Design review of the part built by this model. Coordinates are the model's own, in mm. A direction names the side the tool comes from. Give positions to 0.01 mm unless a question says otherwise; leave off trailing zeros. Write each loop counter-clockwise with the first axis right and the second up, starting at its lowest first coordinate (ties: lowest second). Pieces come first, ordered by that corner, then holes.
Autodesk Inventor part; units mm, degrees
ref_plane "Work Plane1" through (-9.8235, 15.24, 1.6002) normal (0, 1, 0) x (1, 0, 0)
ref_plane "YZ Plane" through (0, 0, 0) normal (1, 0, 0) x (0, 1, 0)
ref_plane "XZ Plane" through (0, 0, 0) normal (0, 1, 0) x (-1, 0, 0)
ref_plane "Work Plane1" through (-9.8235, 15.24, 1.6002) normal (0, 1, 0) x (1, 0, 0)
sketch "Sketch1" plane through (-9.8235, 15.24, 1.6002) normal (0, 1, 0) x (1, 0, 0)
  line L0 (-1.2255, -6.4008) -> (-0.508, -6.4008)
  arc A0 (-1.7335, -5.8928) -> (-1.2255, -6.4008) centre (-1.2255, -5.8928) ccw
  line L1 (-1.7335, 9.0932) -> (-1.7335, -5.8928)
  arc A1 (-0.508, -6.4008) -> (0, -5.8928) centre (-0.508, -5.8928) ccw
  line L2 (0, -5.8928) -> (0, 0)
  line L3 (-1.0858, 9.6012) -> (-1.2256, 9.6012)
  arc A2 (-0.5778, 9.0932) -> (-1.0858, 9.6012) centre (-1.0858, 9.0932) ccw
  line L4 (0, 0) -> (19.6469, 0)
  line L5 (19.6469, 0) -> (19.6469, -5.8928)
  arc A3 (19.6469, -5.8928) -> (20.1549, -6.4008) centre (20.1549, -5.8928) ccw
  line L6 (20.1549, -6.4008) -> (20.8725, -6.4008)
  arc A4 (20.8725, -6.4008) -> (21.3804, -5.8928) centre (20.8725, -5.8928) ccw
  line L7 (21.3804, -5.8928) -> (21.3804, 9.0932)
  arc A5 (21.3804, 9.0932) -> (20.8725, 9.6012) centre (20.8725, 9.0932) ccw
  arc A6 (20.7327, 9.6012) -> (20.2247, 9.0932) centre (20.7327, 9.0932) ccw
  line L8 (20.8725, 9.6012) -> (20.7327, 9.6012)
  line L9 (-0.5778, 9.0932) -> (-0.5778, 3.7084)
  arc A7 (-0.5778, 3.7084) -> (-0.0698, 3.2004) centre (-0.0698, 3.7084) ccw
  line L10 (-0.0698, 3.2004) -> (1.4182, 3.2004)
  arc A8 (1.4182, 3.2004) -> (1.9262, 3.7084) centre (1.4182, 3.7084) ccw
  line L11 (1.9262, 3.7084) -> (1.9262, 9.0932)
  arc A9 (-0.5778, 9.0932) -> (-1.0858, 9.6012) centre (-1.0859, 9.0932) ccw
  arc A10 (-1.2256, 9.6012) -> (-1.7335, 9.0932) centre (-1.2256, 9.0932) ccw
  line L12 (-1.2256, 9.6012) -> (-1.0858, 9.6012)
  arc A11 (2.4342, 9.6012) -> (1.9262, 9.0932) centre (2.4342, 9.0932) ccw
  line L13 (2.4342, 9.6012) -> (2.5739, 9.6012)
  arc A12 (3.0819, 9.0932) -> (2.5739, 9.6012) centre (2.5739, 9.0932) ccw
  line L14 (3.0819, 9.0932) -> (3.0819, 3.7084)
  arc A13 (3.0819, 3.7084) -> (3.5899, 3.2004) centre (3.5899, 3.7084) ccw
  line L15 (3.5899, 3.2004) -> (5.0779, 3.2004)
  arc A14 (5.0779, 3.2004) -> (5.5859, 3.7084) centre (5.0779, 3.7084) ccw
  line L16 (5.5859, 3.7084) -> (5.5859, 9.0932)
  arc A15 (6.0939, 9.6012) -> (5.5859, 9.0932) centre (6.0939, 9.0932) ccw
  line L17 (6.0939, 9.6012) -> (6.2336, 9.6012)
  arc A16 (6.7416, 9.0932) -> (6.2336, 9.6012) centre (6.2336, 9.0932) ccw
  line L18 (6.7416, 9.0932) -> (6.7416, 3.7084)
  arc A17 (6.7416, 3.7084) -> (7.2496, 3.2004) centre (7.2496, 3.7084) ccw
  line L19 (7.2496, 3.2004) -> (8.7376, 3.2004)
  arc A18 (8.7376, 3.2004) -> (9.2456, 3.7084) centre (8.7376, 3.7084) ccw
  line L20 (9.2456, 3.7084) -> (9.2456, 9.0932)
  arc A19 (9.7536, 9.6012) -> (9.2456, 9.0932) centre (9.7536, 9.0932) ccw
  line L21 (9.7536, 9.6012) -> (9.8933, 9.6012)
  arc A20 (10.4013, 9.0932) -> (9.8933, 9.6012) centre (9.8933, 9.0932) ccw
  line L22 (10.4013, 9.0932) -> (10.4013, 3.7084)
  arc A21 (10.4013, 3.7084) -> (10.9093, 3.2004) centre (10.9093, 3.7084) ccw
  line L23 (10.9093, 3.2004) -> (12.3973, 3.2004)
  arc A22 (12.3973, 3.2004) -> (12.9053, 3.7084) centre (12.3973, 3.7084) ccw
  line L24 (12.9053, 3.7084) -> (12.9053, 9.0932)
  arc A23 (13.4133, 9.6012) -> (12.9053, 9.0932) centre (13.4133, 9.0932) ccw
  line L25 (13.4133, 9.6012) -> (13.553, 9.6012)
  arc A24 (14.061, 9.0932) -> (13.553, 9.6012) centre (13.553, 9.0932) ccw
  line L26 (14.061, 9.0932) -> (14.061, 3.7084)
  arc A25 (14.061, 3.7084) -> (14.569, 3.2004) centre (14.569, 3.7084) ccw
  line L27 (14.569, 3.2004) -> (16.057, 3.2004)
  arc A26 (16.057, 3.2004) -> (16.565, 3.7084) centre (16.057, 3.7084) ccw
  line L28 (16.565, 3.7084) -> (16.565, 9.0932)
  arc A27 (17.073, 9.6012) -> (16.565, 9.0932) centre (17.073, 9.0932) ccw
  line L29 (17.073, 9.6012) -> (17.2127, 9.6012)
  arc A28 (17.7207, 9.0932) -> (17.2127, 9.6012) centre (17.2127, 9.0932) ccw
  line L30 (17.7207, 9.0932) -> (17.7207, 3.7084)
  arc A29 (17.7207, 3.7084) -> (18.2287, 3.2004) centre (18.2287, 3.7084) ccw
  line L31 (18.2287, 3.2004) -> (19.7167, 3.2004)
  arc A30 (19.7167, 3.2004) -> (20.2247, 3.7084) centre (19.7167, 3.7084) ccw
  line L32 (20.2247, 3.7084) -> (20.2247, 9.0932)
  dimension "d0" = 21.9583
  dimension "d1" = 3.6597
sketch "Sketch2" plane through (0, 0, 0) normal (0, 1, 0) x (-1, 0, 0)
  line L0 (-9.8235, 1.6002) -> (-9.8235, 7.493)
  arc A0 (-9.8235, 7.493) -> (-10.3314, 8.001) centre (-10.3314, 7.493) ccw
  line L1 (-10.3314, 8.001) -> (-11.049, 8.001)
  arc A1 (-11.049, 8.001) -> (-11.557, 7.493) centre (-11.049, 7.493) ccw
  line L2 (-11.557, 7.493) -> (-11.557, -7.493)
  arc A2 (-11.557, -7.493) -> (-11.049, -8.001) centre (-11.049, -7.493) ccw
  arc A3 (-10.9093, -8.001) -> (-10.4013, -7.493) centre (-10.9093, -7.493) ccw
  line L3 (-10.4013, -2.1082) -> (-10.4013, -7.493)
  arc A4 (-9.8933, -1.6002) -> (-10.4013, -2.1082) centre (-9.8933, -2.1082) ccw
  line L4 (-8.4053, -1.6002) -> (-9.8933, -1.6002)
  line L5 (-11.049, -8.001) -> (-10.9093, -8.001)
  arc A5 (-7.8973, -2.1082) -> (-8.4053, -1.6002) centre (-8.4053, -2.1082) ccw
  line L6 (-7.8973, -7.493) -> (-7.8973, -2.1082)
  arc A6 (-7.8973, -7.493) -> (-7.3893, -8.001) centre (-7.3893, -7.493) ccw
  line L7 (-7.2496, -8.001) -> (-7.3893, -8.001)
  arc A7 (-7.2496, -8.001) -> (-6.7416, -7.493) centre (-7.2496, -7.493) ccw
  line L8 (-6.7416, -2.1082) -> (-6.7416, -7.493)
  arc A8 (-6.2336, -1.6002) -> (-6.7416, -2.1082) centre (-6.2336, -2.1082) ccw
  line L9 (-4.7456, -1.6002) -> (-6.2336, -1.6002)
  arc A9 (-4.2376, -2.1082) -> (-4.7456, -1.6002) centre (-4.7456, -2.1082) ccw
  line L10 (-4.2376, -7.493) -> (-4.2376, -2.1082)
  arc A10 (-4.2376, -7.493) -> (-3.7296, -8.001) centre (-3.7296, -7.493) ccw
  line L11 (-3.5899, -8.001) -> (-3.7296, -8.001)
  arc A11 (-3.5899, -8.001) -> (-3.0819, -7.493) centre (-3.5899, -7.493) ccw
  line L12 (-3.0819, -2.1082) -> (-3.0819, -7.493)
  arc A12 (-2.5739, -1.6002) -> (-3.0819, -2.1082) centre (-2.5739, -2.1082) ccw
  line L13 (-1.0858, -1.6002) -> (-2.5739, -1.6002)
  arc A13 (-0.5778, -2.1082) -> (-1.0858, -1.6002) centre (-1.0858, -2.1082) ccw
  line L14 (-0.5778, -7.493) -> (-0.5778, -2.1082)
  arc A14 (-0.5778, -7.493) -> (-0.0698, -8.001) centre (-0.0698, -7.493) ccw
  line L15 (0.0699, -8.001) -> (-0.0698, -8.001)
  arc A15 (0.0699, -8.001) -> (0.5779, -7.493) centre (0.0699, -7.493) ccw
  line L16 (0.5779, -2.1082) -> (0.5779, -7.493)
  arc A16 (1.0859, -1.6002) -> (0.5779, -2.1082) centre (1.0859, -2.1082) ccw
  line L17 (2.5739, -1.6002) -> (1.0859, -1.6002)
  arc A17 (3.0819, -2.1082) -> (2.5739, -1.6002) centre (2.5739, -2.1082) ccw
  line L18 (3.0819, -7.493) -> (3.0819, -2.1082)
  arc A18 (3.0819, -7.493) -> (3.5899, -8.001) centre (3.5899, -7.493) ccw
  line L19 (3.7296, -8.001) -> (3.5899, -8.001)
  arc A19 (3.7296, -8.001) -> (4.2376, -7.493) centre (3.7296, -7.493) ccw
  line L20 (4.2376, -2.1082) -> (4.2376, -7.493)
  arc A20 (4.7456, -1.6002) -> (4.2376, -2.1082) centre (4.7456, -2.1082) ccw
  line L21 (6.2336, -1.6002) -> (4.7456, -1.6002)
  arc A21 (6.7416, -2.1082) -> (6.2336, -1.6002) centre (6.2336, -2.1082) ccw
  line L22 (6.7416, -7.493) -> (6.7416, -2.1082)
  arc A22 (6.7416, -7.493) -> (7.2496, -8.001) centre (7.2496, -7.493) ccw
  line L23 (7.3893, -8.001) -> (7.2496, -8.001)
  arc A23 (7.3893, -8.001) -> (7.8973, -7.493) centre (7.3893, -7.493) ccw
  line L24 (7.8973, -2.1082) -> (7.8973, -7.493)
  arc A24 (8.4053, -1.6002) -> (7.8973, -2.1082) centre (8.4053, -2.1082) ccw
  line L25 (9.8933, -1.6002) -> (8.4053, -1.6002)
  arc A25 (10.4013, -2.1082) -> (9.8933, -1.6002) centre (9.8933, -2.1082) ccw
  line L26 (10.4013, -7.493) -> (10.4013, -2.1082)
  arc A26 (10.4013, -7.493) -> (10.9093, -8.001) centre (10.9093, -7.493) ccw
  line L27 (10.9093, -8.001) -> (11.049, -8.001)
  arc A27 (11.049, -8.001) -> (11.557, -7.493) centre (11.049, -7.493) ccw
  line L28 (11.557, -7.493) -> (11.557, 7.493)
  arc A28 (11.557, 7.493) -> (11.049, 8.001) centre (11.049, 7.493) ccw
  line L29 (11.049, 8.001) -> (10.3315, 8.001)
  arc A29 (10.3315, 8.001) -> (9.8235, 7.493) centre (10.3315, 7.493) ccw
  line L30 (9.8235, 7.493) -> (9.8235, 1.6002)
  line L31 (9.8235, 1.6002) -> (-9.8235, 1.6002)
  point P0 (0, 0)
extrude "Extrusion1" add sketch "Sketch2" along normal blind 30.5
sketch "Sketch3" plane through (0, 0, 0) normal (0, -1, 0) x (1, 0, 0)
  line L0 (-9.8235, 1.6002) -> (9.8235, 1.6002) construction
  circle A0 centre (9.05, -0.3998) radius 0.75
  circle A1 centre (-9.05, -0.3998) radius 0.75
  line L1 (9.05, -0.3998) -> (0, 0) construction
  line L2 (0, 0) -> (-9.05, -0.3998) construction
  dimension "d11" = 1.5
  dimension "d12" = 2
  dimension "d13" = 18.1
extrude "Extrusion2" add sketch "Sketch3" along normal blind 3.6
equation "\"d1\" = 0.166667 * d0"
properties part number "WA-T247-101E"
(1) Consider section A-A, the plane z = -6. Give the boundary of the cut face in (x, y), then the cut area to 3 significant figures.
Resolved:
outline: (-11.56, 0) - (-10.4, 0) - (-10.4, 30.5) - (-11.56, 30.5) - close; (-7.9, 0) - (-6.74, 0) - (-6.74, 30.5) - (-7.9, 30.5) - close; (-4.24, 0) - (-3.08, 0) - (-3.08, 30.5) - (-4.24, 30.5) - close; (-0.58, 0) - (0.58, 0) - (0.58, 30.5) - (-0.58, 30.5) - close; (3.08, 0) - (4.24, 0) - (4.24, 30.5) - (3.08, 30.5) - close; (6.74, 0) - (7.9, 0) - (7.9, 30.5) - (6.74, 30.5) - close; (10.4, 0) - (11.56, 0) - (11.56, 30.5) - (10.4, 30.5) - close
area: 247 mm2
(2) Consider section C-C, the plane x = 9.05. Give the boundary of the cut face in (y, z).
Resolved:
outline: (-3.6, -1.15) - (0, -1.15) - (0, -1.6) - (30.5, -1.6) - (30.5, 1.6) - (0, 1.6) - (0, 0.35) - (-3.6, 0.35) - close
(3) Clearance check with flat-ended pins moving along their axes: P1, Ø1.2, axis at x = -5.5, y = 23, coming from the -Z side; P2, Ø5, axis at x = 5.5, z = -3.5, coming from the -Y side; P3, Ø3, axis at x = 5, y = 4, coming from the +Z side. State where each tip first meets the part, or that it passes through.
Resolved:
P1: stops at z = -1.6
P2: stops at y = 0
P3: stops at z = 1.6
(4) To check wall thickness, follow L1, parallel to X at y = 1, z = 3.5; L2, parallel to Z at x = 5, y = 25; L3, parallel to Y at x = 4.5, z = -1. State the ranges of each line that lie inside material, in increasing order.
Resolved:
L1: x = -11.56 to -9.82, 9.82 to 11.56
L2: z = -1.6 to 1.6
L3: y = 0 to 30.5
(5) Tool access review of faces 1 (the face through (2, 15, -1.6)), 2 (the face through (-8.335, -1.775, -0.625)), 3 (the face through (-11.557, 15, 0)), 4 (the face through (9.824, 15, 5)): name each direction out of +Z, -Z, +X, -X, +Y, -Y from which nothing blocks a thin tool from reaching the whole face with its end or side.
Resolved:
face 1: -Z, +Y, -Y
face 2: -Y
face 3: +Z, -Z, -X, +Y, -Y
face 4: +Z, +Y, -Y
(6) Consider section B-B, the plane z = 3.5. Give the boundary of the cut face in (x, y).
Resolved:
outline: (-11.56, 0) - (-9.82, 0) - (-9.82, 30.5) - (-11.56, 30.5) - close; (9.82, 0) - (11.56, 0) - (11.56, 30.5) - (9.82, 30.5) - close
